Can you work these out from the model? Positions are in its coordinate system, mm. A direction names the side the tool comes from. Give positions to 0.01 mm unless a question says otherwise; leave off trailing zeros. Order: outer loops, then holes, each group sorted by start corner. A loop starts at its lowest first (then second) coordinate and runs counter-clockwise, first axis right, second up. Notation, with made-up numbers: (-35, -14.75) - (-30, -14.75) arc R9 cw to (-30, 2.25) - close; hole circle Ø4 at (61.25, 13). An arc over 180 degrees is marked (long way). Answer as CSV lines item,"result".
```python
from build123d import *

# Parameters (mm, degrees)
SKETCH044_R           = 32.5
PAD022_DEPTH          = 10
THICKNESS002_T        = -2.4
PAD023_DEPTH          = 5
POLARPATTERN012_COUNT = 6


with BuildPart() as part:
    # Sketch044 → Pad022 (new body)
    with BuildSketch(Plane.XY):
        Circle(SKETCH044_R)
    extrude(amount=PAD022_DEPTH)

    # Thickness002
    thickness002_openings = [part.faces().sort_by_distance(p)[0] for p in [
        (0, 0, 0),
    ]]
    offset(amount=THICKNESS002_T, openings=thickness002_openings)

    # Sketch045 (on Face2 of Pad022) → Pad023 (join)
    with BuildSketch(Plane(origin=(0, 0, 0), x_dir=(1, 0, 0), z_dir=(0, 0, -1))):
        with BuildLine():
            Line((-7, 31.7372021451), (-7, 29.1719042916))
            ThreePointArc((7, 29.1719042916), (0, 30), (-7, 29.1719042916))
            Line((7, 29.1719042916), (7, 31.7372021451))
            ThreePointArc((7, 31.7372021451), (0, 32.5), (-7, 31.7372021451))
        make_face()
    pad023 = extrude(amount=PAD023_DEPTH)

    # PolarPattern012: Pad023 ×6 about axis
    polarpattern012_axis = Axis((0, 0, 0), (0, 0, -1))
    for i in range(1, POLARPATTERN012_COUNT):
        add(pad023.rotate(polarpattern012_axis, i * 360 / POLARPATTERN012_COUNT))


solid = part.part
```
1) I'm going to push flat-ended pins straight in: P1, Ø8, axis at x = 9, y = -9.5, coming from the -Z side; P2, Ø1.3, axis at y = 30, z = -2.5, coming from the +X side; P3, Ø1.5, axis at y = -24, z = -2.5, coming from the +X side; P4, Ø3, axis at x = 30.5, y = -4, coming from the -Z side. Where does each tip first touch, or does it pass through?
Answer block:
P1,"z = 7.6"
P2,"x = 7"
P3,"through"
P4,"z = 0"
2) I want a section at C-C on z = 1.75. Write out the boundary of the cut face in (x, y), plus the area to 3 significant figures.
Answer block:
outline,"circle Ø65 at (0, 0); hole circle Ø60.2 at (0, 0)"
area,"472 mm2"
3) I need wall thicknesses on line 1 along X through (y, z) = (0, 2.75); line 2 along Z through (x, y) = (4.5, -3.5). Which ranges of each line are inside material? Lowest first, please. Write a range as [from, to].
Answer block:
line 1,"[-32.5, -30.1], [30.1, 32.5]"
line 2,"[7.6, 10]"
4) Which directions (+Z, -Z, +X, -X, +Y, -Y) give clear straight access to the entire face, cutting with the end or side of a thin tool? Please do faces 1 (the flat face through (-29.89, -9.174, -2.465)), 2 (the cylindrical face through (-6.525, -29.384, 3.747)), 3 (the cylindrical face through (25.93, 15.09, -2.46)), 4 (the flat face through (-7, 30, -2)).
Answer block:
face 1,"-Z, -X"
face 2,"none"
face 3,"-Z"
face 4,"-Z, -X, +Y, -Y"
5) I want a section at B-B on y = 0. Write out the boundary of the cut face in (x, z), plus the area to 3 significant figures.
Answer block:
outline,"(-32.5, 0) - (-30.1, 0) - (-30.1, 7.6) - (30.1, 7.6) - (30.1, 0) - (32.5, 0) - (32.5, 10) - (-32.5, 10) - close"
area,"192 mm2"
6) I want a section at D-D on z = 9.25. Write out the boundary of the cut face in (x, y), plus the area to 3 significant figures.
Answer block:
outline,"circle Ø65 at (0, 0)"
area,"3,320 mm2"
7) If we mould it in two halves opening along X, with no side actions, what happens to faces 5 (the flat face through (22.89, -21.3, -2.46)), 6 (the flat face through (-29.859, 9.156, -2.465)), 7 (the flat face through (31, 0, 0))? For each: +X half, -X half, draft (parallel to the pull), parting line (faces both ways), or undercut.
Answer block:
face 5,"undercut"
face 6,"-X half"
face 7,"draft"
8) I want a section at A-A on x = 0. Write out the boundary of the cut face in (y, z), plus the area to 3 significant figures.
Answer block:
outline,"(-32.5, -5) - (-30, -5) - (-30, 0) - (-30.1, 0) - (-30.1, 7.6) - (30.1, 7.6) - (30.1, 0) - (30, 0) - (30, -5) - (32.5, -5) - (32.5, 10) - (-32.5, 10) - close"
area,"217 mm2"
